Geometry: final body of the model. Coordinates: model frame, mm. Face numbers are marked on the shaded views. A direction names the side the tool comes from. Coordinates: 2 decimals unless noted, no trailing zeros. Write each loop counter-clockwise with the first axis right and the second up, starting at its lowest first coordinate (ties: lowest second). Pieces come first, ordered by that corner, then holes. Notation, with made-up numbers: (28.25, 61.25) - (51.25, 61.25) arc R12 ccw to (51.25, 67.25) - close; hole circle Ø11 at (82.25, -15.5). An arc over 180 degrees is marked (long way). Answer as a JSON object with one key per item and string values. Group by question number.
Item 1: Section C-C on x = 0. Return loops of the section in (y, z).
Item 2: Set-up query: the marked faces 5, 6 and 7. Return all of +Z, -Z, +X, -X, +Y, -Y with unobstructed straight access to the full face (end or side cutting, diameter ignored); none if empty.
Item 3: First-contact query: pin 1 Ø2.5 at (y, z) = (-44.5, 4) entering from -X; pin 2 Ø2.5 at (y, z) = (-42, 2.5) entering from -X; pin 3 Ø2.5 at (y, z) = (-42, 3.5) entering from +X; pin 4 Ø12 at (x, y) = (6.5, -32.5) entering from -Z. Flat tips, straight axial feed; report the tip coordinate or a pass-through.
Item 4: Line query: line 1 along X through (y, z) = (-12.5, 2.25); line 2 along X through (y, z) = (1, 0.95); line 3 along Y through (x, z) = (-56.5, 5.05). Output: solid intervals per line, ascending. Write a range as from..to.
Item 5: Section A-A on y = 2. Return loops of the section in (x, z), and give its area (3 significant figures).
Item 6: Mould query, pull axis Y, two halves, no side actions, for the marked faces 1, 2, 3 and 4. Classes: pulls with the +Y half, pulls with the -Y half, needs draft (parallel to the pull), parting line crosses it, or undercut.
Item 7: Section B-B on x = -38.5. Return loops of the section in (y, z).
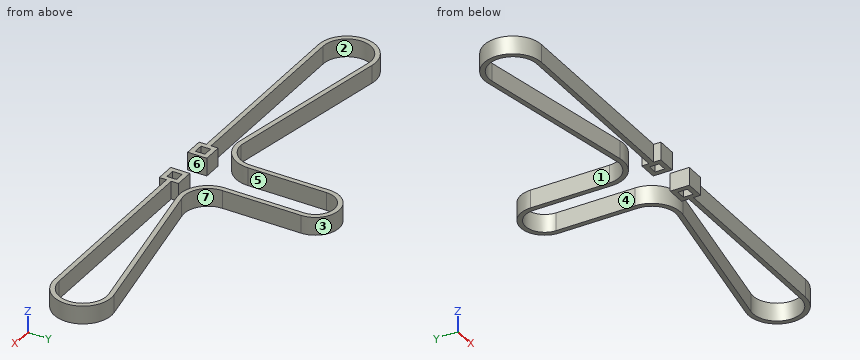
```python
from build123d import *

# Parameters (mm, degrees)
F0_W     = 3.175
F0_H     = 3.175
F1_DEPTH = 6


with BuildPart() as f1:
    # F0 (on Top) → F1 (new body)
    with BuildSketch(Plane.XY):
        with BuildLine():
            Line((-6.35, -26.23185), (-6.35, 0))
            ThreePointArc((-6.35, 0), (0, 6.35), (6.35, 0))
            Line((6.35, 0), (6.35, -26.23185))
            ThreePointArc((6.35, -26.23185), (9.777239, -33.549154), (17.59261, -35.600705))
            Line((17.59261, -35.600705), (72.315666, -25.568221))
            ThreePointArc((72.315666, -25.568221), (81.651911, -32.656978), (73.747008, -41.3131))
            Line((73.747008, -41.3131), (11.1125, -41.3131))
            Line((11.1125, -41.3131), (11.1125, -42.9006))
            Line((11.1125, -42.9006), (73.747008, -42.9006))
            ThreePointArc((73.747008, -42.9006), (83.232933, -32.513714), (72.030307, -24.006578))
            Line((72.030307, -24.006578), (17.59261, -33.981284))
            ThreePointArc((17.59261, -33.981284), (10.906581, -32.422062), (7.9375, -26.23185))
            Line((7.9375, -26.23185), (7.9375, 0))
            ThreePointArc((7.9375, 0), (0, 7.9375), (-7.9375, 0))
            Line((-7.9375, 0), (-7.9375, -26.23185))
            ThreePointArc((-7.9375, -26.23185), (-10.26234, -31.84451), (-15.875, -34.16935))
            Line((-15.875, -34.16935), (-72.05076, -24.002854))
            ThreePointArc((-72.05076, -24.002854), (-83.233868, -32.524067), (-73.747008, -42.9006))
            Line((-73.747008, -42.9006), (-11.1125, -42.9006))
            Line((-11.1125, -42.9006), (-11.1125, -41.3131))
            Line((-11.1125, -41.3131), (-73.747008, -41.3131))
            ThreePointArc((-73.747008, -41.3131), (-81.651911, -32.656978), (-72.315666, -25.568221))
            Line((-72.315666, -25.568221), (-17.59261, -35.600705))
            ThreePointArc((-17.59261, -35.600705), (-9.777239, -33.549154), (-6.35, -26.23185))
        make_face()
        Polygon((-11.1125, -38.93185), (-11.1125, -41.3131), (-11.1125, -42.9006), (-11.1125, -45.28185), (-4.7625, -45.28185), (-4.7625, -38.93185), align=None)
        with Locations((-7.9375, -42.10685)):
            Rectangle(F0_W, F0_H, mode=Mode.SUBTRACT)
        Polygon((11.1125, -42.9006), (11.1125, -41.3131), (11.1125, -38.93185), (4.7625, -38.93185), (4.7625, -45.28185), (11.1125, -45.28185), align=None)
        with Locations((7.9375, -42.10685)):
            Rectangle(F0_W, F0_H, mode=Mode.SUBTRACT)
    extrude(amount=F1_DEPTH)


solid = f1.part
```
Checks:
{
 "1": {"outline": "(6.35, 0) - (7.94, 0) - (7.94, 6) - (6.35, 6) - close"},
 "2": {"face 5": "+Z, -Z", "face 6": "+Z, -Z, -Y", "face 7": "+Z, -Z, +Y"},
 "3": {"pin 1": "x = -11.11", "pin 2": "x = -79.78", "pin 3": "x = 79.78", "pin 4": "z = 0"},
 "4": {"line 1": "-7.94..-6.35, 6.35..7.94", "line 2": "-7.87..-6.27, 6.27..7.87", "line 3": "-42.9..-41.31, -28.47..-26.82"},
 "5": {"outline": "(-7.68, 0) - (-6.03, 0) - (-6.03, 6) - (-7.68, 6) - close; (6.03, 0) - (7.68, 0) - (7.68, 6) - (6.03, 6) - close", "area": "19.9 mm^2"},
 "6": {"face 1": "needs draft", "face 2": "undercut", "face 3": "pulls with the +Y half", "face 4": "undercut"},
 "7": {"outline": "(-42.9, 0) - (-41.31, 0) - (-41.31, 6) - (-42.9, 6) - close; (-31.77, 0) - (-30.07, 0) - (-30.07, 6) - (-31.77, 6) - close"}
}
